Design review of the part built by this model. Coordinates are the model's own, in mm. A direction names the side the tool comes from. Give positions to 0.01 mm unless a question says otherwise; leave off trailing zeros. Write each loop counter-clockwise with the first axis right and the second up, starting at its lowest first coordinate (ties: lowest second). Pieces come first, ordered by that corner, then holes. Notation, with made-up numbers: M 27,-5.5 L 39,-5.5 A18 cw 39,16.5 Z; hole C 48,34.5 d1. An arc over 180 degrees is marked long. Use a Markdown table: item, result. Add a question column.
```python
from build123d import *

# Parameters (mm, degrees)
EXTRUDE_1_DEPTH           = 388.6
HOLE_WIZARD_1_D           = 4
HOLE_WIZARD_1_CBORE_D     = 7
HOLE_WIZARD_1_CBORE_DEPTH = 3.5


with BuildPart() as part:
    # 草图1 → 凸台-拉伸1 (new body)
    with BuildSketch(Plane.XY):
        Polygon((0, 16.475), (0, -16.475), (6.5, -16.475), (6.5, -2), (10, -2), (10, 2), (6.5, 2), (6.5, 16.475), align=None)
    extrude(amount=EXTRUDE_1_DEPTH)

    # 打孔尺寸(%根据)内六角圆柱头螺钉的类型1 (through all)
    with Locations(Plane(origin=(6.5, 0, 0), x_dir=(0, 0, -1), z_dir=(1, 0, 0))):
        with Locations((-382.6, -7.5), (-364.6, -7.5), (-364.6, 7.5), (-382.6, 7.5), (-24, 7.5), (-24, -7.5), (-6, -7.5), (-6, 7.5)):
            CounterBoreHole(HOLE_WIZARD_1_D / 2, HOLE_WIZARD_1_CBORE_D / 2, HOLE_WIZARD_1_CBORE_DEPTH)


solid = part.part
```
(1) For pin 1 (4.5 mm diameter, centred on y = 7.5, z = 382.6, fed in from -X); pin 2 (1.8 mm diameter, centred on x = 8.5, z = 285, fed in from +Y); pin 3 (4.5 mm diameter, centred on y = -7.5, z = 364.6, fed in from +X); pin 4 (5.5 mm diameter, centred on y = 7, z = 366, fed in from +X), all flat-tipped, find the tip position at first contact; note any pin that passes through.
(2) Add section A-A on z = 208. Give the boundary of the cut face in (x, y) (3 decimals).
(3) The part is to be moulded in two halves that separate along Z. For faces 1 (the flat face through (4, 0, 0)), 2 (the cylindrical face through (4.77, 8.55, 379.26)), 3 (the flat face through (3, 16.475, 192)), 4 (the flat face through (3, -9, 22)), say which applies: released by +Z, released by -Z, zero draft, split by the parting line, or undercut.
(4) Wall thickness on L1, parallel to Y at x = 2, z = 6 (3 decimals); L2, parallel to Y at x = 5.1, z = 24 (3 decimals); L3, parallel to Z at x = 3.75, y = -5: over which ranges is each line inside the solid? List them lowest first.
(5) Machinability: for faces 5 (the flat face through (3, -16.475, 192)), 6 (the flat face through (6.5, 9, 192)), 7 (the cylindrical face through (4.77, -6.45, 361.26)), which of the approach directions +Z, -Z, +X, -X, +Y, -Y give a long, thin tool a straight path to every point of the face, cutting with its end or side? Answer none if there is none.
From the geometry:
| question | item | result |
|---|---|---|
| 1 | pin 1 | stops at x = 0 |
| 1 | pin 2 | stops at y = 2 |
| 1 | pin 3 | stops at x = 3 |
| 1 | pin 4 | stops at x = 6.5 |
| 2 | outline | M 0,-16.475 L 6.5,-16.475 L 6.5,-2 L 10,-2 L 10,2 L 6.5,2 L 6.5,16.475 L 0,16.475 Z |
| 3 | face 1 | released by -Z |
| 3 | face 2 | undercut |
| 3 | face 3 | zero draft |
| 3 | face 4 | undercut |
| 4 | L1 | y = -16.475 to -9.5, -5.5 to 5.5, 9.5 to 16.475 |
| 4 | L2 | y = -16.475 to -11, -4 to 4, 11 to 16.475 |
| 4 | L3 | z = 0 to 3.55, 8.45 to 21.55, 26.45 to 362.15, 367.05 to 380.15, 385.05 to 388.6 |
| 5 | face 5 | +Z, -Z, +X, -X, -Y |
| 5 | face 6 | +Z, -Z, +X, +Y |
| 5 | face 7 | +X |
